Can you work these out from the drawing? Everything is in mm from the part's minimum corner. A direction names the side the tool comes from. Coordinates: 2 decimals unless noted, no trailing zeros. Loops run counter-clockwise (first coordinate to the right, second up) from the corner with the lowest first, then second, coordinate; pieces in that order, holes last. Notation, with made-up numbers: (-34.75, -21.75) -> (-5.75, -21.75) arc R15 cw to (-5.75, -13.75) -> close; hole circle Ø11 at (-10.75, 42). An arc over 180 degrees is marked (long way). Put each result on its own line as item: value. Start each with the question number.
Item 1: For the marked faces 5, 6 and 7, which set-ups out of +Z, -Z, +X, -X, +Y, -Y let a thin tool reach every point of the face, with its end or its side?
Item 2: If we section it at B-B on x = 30: Please give me the cut outline in (y, z).
Item 3: Will these pins go through, and if not, where does the flat tip stop? P1, Ø6, axis at y = 22.5, z = 7.5, coming from the +X side; P2, Ø1, axis at x = 13.5, z = 8, coming from the +Y side; P3, Ø2.5, axis at x = 41, z = 10, coming from the +Y side.
Item 4: If we section it at A-A on y = 21.5: Please give me the cut outline in (x, z).
Item 5: Please list where these lines run through material, in increasing order: L1, parallel to X at y = 12, z = 14.5; L2, parallel to X at y = 41.5, z = 10; L3, parallel to Z at x = 41, y = 40.5. Write a range as from..to.
Item 6: We'd pull the mould along X, two halves only. Please class the marked faces 1, 2, 3 and 4: pulls with the +X half, pulls with the -X half, needs draft (parallel to the pull), parting line crosses it, or undercut.
Item 7: If we section it at D-D on z = 14: Please give me the cut outline in (x, y), plus the area to 3 significant figures.
Item 8: If we section it at C-C on x = 41: Please give me the cut outline in (y, z), plus the area to 3 significant figures.
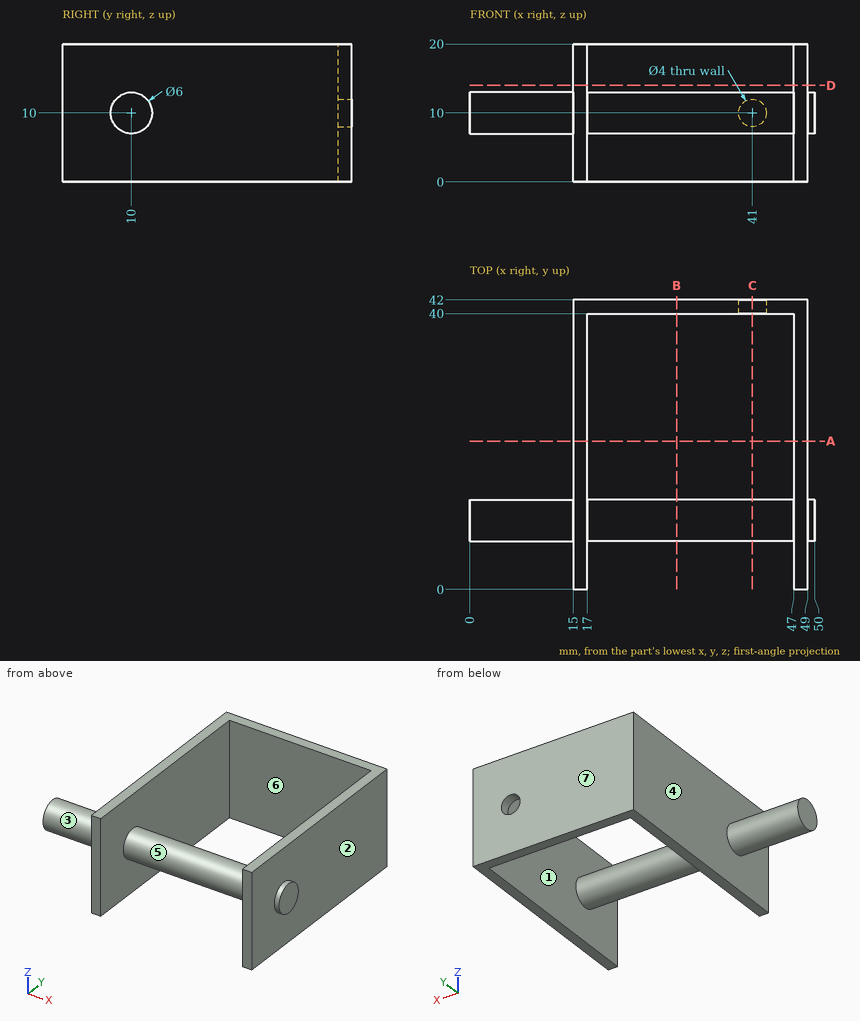
Solutions:
1. face 5: none
1. face 6: +Z, -Z
1. face 7: +Z, -Z, +X, -X, +Y
2. outline: circle Ø6 at (10, 10); (40, 0) -> (42, 0) -> (42, 20) -> (40, 20) -> close
3. P1: x = 49
3. P2: y = 12.6
3. P3: y = 13
4. outline: (15, 0) -> (17, 0) -> (17, 20) -> (15, 20) -> close; (47, 0) -> (49, 0) -> (49, 20) -> (47, 20) -> close
5. L1: 15..17, 47..49
5. L2: 15..39, 43..49
5. L3: 0..8, 12..20
6. face 1: undercut
6. face 2: pulls with the +X half
6. face 3: needs draft
6. face 4: pulls with the -X half
7. outline: (15, 0) -> (17, 0) -> (17, 40) -> (47, 40) -> (47, 0) -> (49, 0) -> (49, 42) -> (15, 42) -> close
7. area: 228 mm^2
8. outline: circle Ø6 at (10, 10); (40, 0) -> (42, 0) -> (42, 8) -> (40, 8) -> close; (40, 12) -> (42, 12) -> (42, 20) -> (40, 20) -> close
8. area: 60.3 mm^2
